from build123d import *

# Parameters (mm, degrees)
F0_W     = 113.2690608501
F0_H     = 86.9128275663
F2_DEPTH = 25.4
F3_DEPTH = 25.4
F4_T     = -2.54


# Not quite as in the source:
# - a feature names something its author has since deleted; it is built from what else it names
# - the program builds the solid bodies; features that only make, move or delete a surface that nothing else refers to are left out


with BuildPart() as f2:
    # F0 (on Front) → F2 (new body)
    with BuildSketch(Plane.XZ):
        with Locations((-9.0991780162, 12.3919239268)):
            Rectangle(F0_W, F0_H)
    extrude(amount=F2_DEPTH)

    # F3 (add): a face of the model
    f3_faces = [f2.faces().sort_by_distance(p)[0] for p in [
        (-9.0991780162, -25.4, 12.3919239268),
    ]]
    extrude(f3_faces, amount=F3_DEPTH)

    # F4
    f4_openings = [f2.faces().sort_by_distance(p)[0] for p in [
        (-9.099178, 0, 12.391924),
    ]]
    offset(amount=F4_T, openings=f4_openings)


with BuildPart() as f2_1:
    # F10: moved
    add(f2.part)


solid = f2_1.part
Design review of the part built by this model. Coordinates are the model's own, in mm. A direction names the side the tool comes from. Round coordinates to 2 decimals unless told otherwise and drop trailing zeros. Loops run counter-clockwise (first coordinate to the right, second up) from the corner with the lowest first, then second, coordinate; pieces in that order, holes last. Notation, with made-up numbers: (-18, -31.5) -> (40, -31.5) arc R14 cw to (40, -9.5) -> close; hole circle Ø9 at (88.5, -16). An arc over 180 degrees is marked (long way). Use one line per item in the form item = value. Start each with the question number.
Q1. Draft analysis for pull direction Z (two halves, no side actions). For faces 1 (the face through (-14, 0, -29)), 2 (the face through (-63.194, -24, 12)), 3 (the face through (-10, -25, -31.064)), state which applies: +Z half, -Z half, draft (parallel to the pull), parting line (faces both ways), or undercut.
Q2. We need section C-C on z = -3. Give the boundary of the cut face in (x, y).
Q3. For pin 1 Ø10 at (x, z) = (-28.5, 13) entering from +Y, flat-tipped, find the tip position at first contact; note if it passes through.
Q4. We need section A-A on x = 10. Give the boundary of the cut face in (y, z).
Q5. Machinability: for faces 4 (the face through (-10, -50.8, 13)), 5 (the face through (44.995, -24, 12)), which of the approach directions +Z, -Z, +X, -X, +Y, -Y give a long, thin tool a straight path to every point of the face, cutting with its end or side? Answer none if there is none.
Q6. We need section B-B on y = -22.5. Give the boundary of the cut face in (x, z).
Q7. Wall thickness on line 1 along X through (y, z) = (-11.5, 47.5); line 2 along Z through (x, y) = (28.5, -11); line 3 along Y through (x, z) = (28, -25.5): over which ranges is each line inside the solid? List them lowest first. Write a range as [from, to].
Calculated:
q1.face_1 = draft
q1.face_2 = undercut
q1.face_3 = -Z half
q2.outline = (-65.73, -50.8) -> (47.54, -50.8) -> (47.54, 0) -> (45, 0) -> (45, -48.26) -> (-63.19, -48.26) -> (-63.19, 0) -> (-65.73, 0) -> close
q3.pin_1 = -48.26
q4.outline = (-50.8, -31.06) -> (0, -31.06) -> (0, -28.52) -> (-48.26, -28.52) -> (-48.26, 53.31) -> (0, 53.31) -> (0, 55.85) -> (-50.8, 55.85) -> close
q5.face_4 = +Z, -Z, +X, -X, -Y
q5.face_5 = +Y
q6.outline = (-65.73, -31.06) -> (47.54, -31.06) -> (47.54, 55.85) -> (-65.73, 55.85) -> close; hole (-63.19, -28.52) -> (45, -28.52) -> (45, 53.31) -> (-63.19, 53.31) -> close
q7.line_1 = [-65.73, -63.19], [45, 47.54]
q7.line_2 = [-31.06, -28.52], [53.31, 55.85]
q7.line_3 = [-50.8, -48.26]
